Input: dimensioned drawing with shaded views. Units: mm. Origin: part minimum x, y, z. Give positions to 0.01 mm unless a question says otherwise; leave off trailing zeros. Order: outer loops, then holes, each group sorted by start corner. A loop starts at its lowest first (then second) coordinate and runs counter-clockwise, first axis right, second up. Notation, with made-up numbers: (33.25, 35) -> (87.25, 35) arc R17 cw to (87.25, 53) -> close; hole circle Ø7 at (38, -28). An arc over 180 degrees is marked (long way). One line per question, with ' | ' between items. Start each with the question number.
(1) Ray query, L1, parallel to Z at x = 114, y = 28; L2, parallel to X at y = 24, z = 5.5; L3, parallel to X at y = 3, z = 8. Return the intervals inside material, ascending.
(2) Section D-D (x = 78). Return loops of the section in (y, z) (3 decimals).
(3) Mould query, pull axis X, two halves, no side actions, for the marked faces 1, 2 and 3. Classes: +X half, -X half, draft (parallel to the pull), parting line (faces both ways), or undercut.
(4) Section C-C (y = 8.5). Return loops of the section in (x, z) (3 decimals).
(5) Section B-B (x = 12.7). Return loops of the section in (y, z) (3 decimals).
(6) Section A-A (z = 6.35). Return loops of the section in (x, y) (3 decimals).
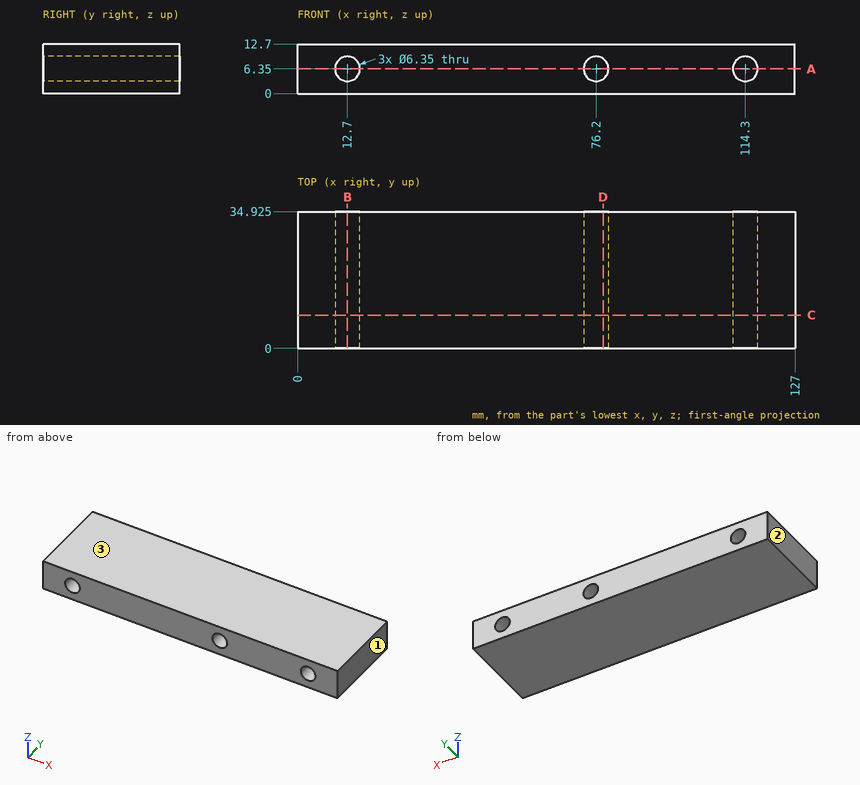
Response:
1) L1: z = 0 to 3.19, 9.51 to 12.7 | L2: x = 0 to 9.64, 15.76 to 73.14, 79.26 to 111.24, 117.36 to 127 | L3: x = 0 to 9.99, 15.41 to 73.49, 78.91 to 111.59, 117.01 to 127
2) outline: (0, 0) -> (34.925, 0) -> (34.925, 3.735) -> (0, 3.735) -> close; (0, 8.965) -> (34.925, 8.965) -> (34.925, 12.7) -> (0, 12.7) -> close
3) face 1: +X half | face 2: -X half | face 3: draft
4) outline: (0, 0) -> (127, 0) -> (127, 12.7) -> (0, 12.7) -> close; hole circle Ø6.35 at (12.7, 6.35); hole circle Ø6.35 at (76.2, 6.35); hole circle Ø6.35 at (114.3, 6.35)
5) outline: (0, 0) -> (34.925, 0) -> (34.925, 3.175) -> (0, 3.175) -> close; (0, 9.525) -> (34.925, 9.525) -> (34.925, 12.7) -> (0, 12.7) -> close
6) outline: (0, 0) -> (9.525, 0) -> (9.525, 34.925) -> (0, 34.925) -> close; (15.875, 0) -> (73.025, 0) -> (73.025, 34.925) -> (15.875, 34.925) -> close; (79.375, 0) -> (111.125, 0) -> (111.125, 34.925) -> (79.375, 34.925) -> close; (117.475, 0) -> (127, 0) -> (127, 34.925) -> (117.475, 34.925) -> close
